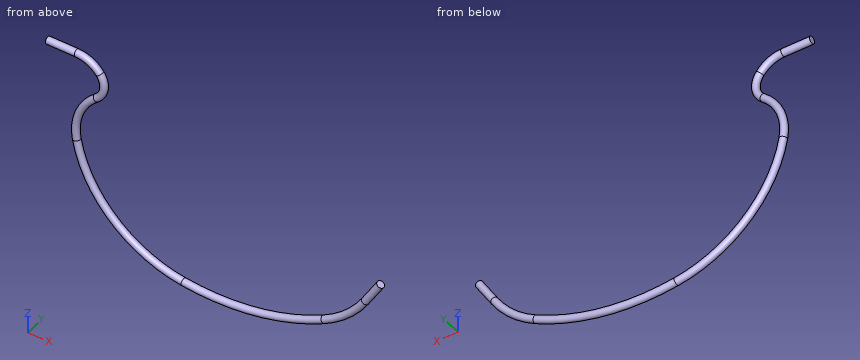
from build123d import *

# Parameters (mm, degrees)
SKETCH_1_R = 2.5


with BuildPart() as part:
    # Wire 2: sweep along a path in SWireLine
    with BuildLine(Plane(origin=(0, 0, 0), x_dir=(1, 0, 0), z_dir=(0, 1, 0))) as wire_2_path:
        Line((0, 0), (20, 0))
        ThreePointArc((20, 0), (29.011943233, 2.091873975), (36.180904523, 7.939698492))
        ThreePointArc((36.180904523, 7.939698492), (38.86499133, 17.80029249), (33.79043443, 26.670721354))
        ThreePointArc((33.79043443, 26.670721354), (21.82641851, 42.786838621), (20, 62.775112886))
        ThreePointArc((20, 62.775112886), (45.584965842, 109.96543175), (94.022959085, 133.101496287))
        ThreePointArc((94.022959085, 133.101496287), (144.087790428, 131.993629879), (191.475888414, 115.804656017))
        ThreePointArc((191.475888414, 115.804656017), (207.587532964, 104.423854927), (220.163330814, 89.226584382))
        Line((220.163330814, 89.226584382), (230.770585075, 72.271167635))
    # 草图1 → Wire 2 (sweep)
    with BuildSketch(Plane(origin=(0, 0, 0), x_dir=(0, 0, -1), z_dir=(1, 0, 0))):
        Circle(SKETCH_1_R)
    sweep(path=wire_2_path.line)


solid = part.part
Build history of the part. All positions in model axes, mm. Round coordinates to 2 decimals unless told otherwise and drop trailing zeros. Loops run counter-clockwise (first coordinate to the right, second up) from the corner with the lowest first, then second, coordinate; pieces in that order, holes last. Notation, with made-up numbers: (-3.75, 75.25) -> (30.25, 75.25) arc R22 ccw to (30.25, 112.25) -> close; hole circle Ø7 at (-8, 9.5). An arc over 180 degrees is marked (long way). Use CSV: the item, a comma, the result in double quotes. Start each with the question number.
Q1. Saw through at B-B on x = 14.5. Give the cut face in (y, z).
Q2. Drill centre lines: L1, parallel to X at y = -0.6, z = -82; L2, parallel to X at y = 0.4, z = -99; L3, parallel to X at y = 0.05, z = -61. Where is each one in solid material? Low to high.
Q3. Flat gauge pins, fed straight in: pin 1 Ø1.5 at (y, z) = (-0.5, -69.5) entering from +X; pin 2 Ø3 at (x, y) = (187.5, 1) entering from -Z; pin 3 Ø2 at (y, z) = (-1.5, -80.5) entering from +X. Where does each tip first touch, or does it go through?
Q4. Saw through at A-A on y = 0. Give the cut face in (x, z), and give its area (3 significant figures).
Solutions:
1,outline,"circle Ø5 at (0, 0)"
2,L1,"x = 23.27 to 28.58, 221.82 to 227.55"
2,L2,"x = 32.78 to 38.95, 209.54 to 216.13"
2,L3,"x = 17.2 to 22.24"
3,pin 1,"stops at x = 24.3"
3,pin 2,"stops at z = -121.22"
3,pin 3,"stops at x = 228.87"
4,outline,"(0, -2.5) -> (20, -2.5) arc R17.96 cw to (34.2, -9.47) arc R10.85 cw to (32.26, -24.69) arc R39.62 ccw to (17.54, -63.23) arc R89.35 ccw to (93.7, -135.58) arc R166.22 ccw to (192.64, -118.02) arc R77.29 ccw to (222.28, -90.55) -> (232.89, -73.6) -> (228.65, -70.95) -> (218.04, -87.9) arc R72.29 cw to (190.32, -113.59) arc R161.22 cw to (94.35, -130.62) arc R84.35 cw to (22.46, -62.32) arc R34.62 cw to (35.32, -28.65) arc R15.85 ccw to (38.16, -6.41) arc R22.96 ccw to (20, 2.5) -> (0, 2.5) -> close"
4,area,"1,850 mm^2"
